```python
from build123d import *

# Parameters (mm, degrees)
BOSS_EXTRUDE1_DEPTH = 2.6
SKETCH3_R           = 1.7
SKETCH3_R_2         = 0.75
BOSS_EXTRUDE2_DEPTH = 4.4
CUT_EXTRUDE1_DEPTH  = 48.070691518
LPATTERN1_COUNT     = 6
LPATTERN1_PITCH     = 8
SKETCH4_R           = 1.95
CUT_EXTRUDE2_DEPTH  = 47.754785851
SKETCH6_W           = 2.6
SKETCH6_H           = 3.6
SKETCH6_W_2         = 4.3
SKETCH6_H_2         = 2.6
BOSS_EXTRUDE4_DEPTH = 1.8
SKETCH7_W           = 2.6
SKETCH7_H           = 1.6
SKETCH7_W_2         = 1.6
SKETCH7_H_2         = 2.6
BOSS_EXTRUDE5_DEPTH = 2
BOSS_EXTRUDE6_START = -2.6
BOSS_EXTRUDE6_DEPTH = 2.6
SKETCH9_R           = 8.5
SKETCH9_R_2         = 4.3
BOSS_EXTRUDE7_DEPTH = 4
SKETCH12_R          = 0.95
CUT_EXTRUDE3_DEPTH  = 4
SKETCH13_W          = 11.452487144
SKETCH13_H          = 18.554951014
SKETCH13_W_2        = 15.080629567
SKETCH13_H_2        = 21.043729538
CUT_EXTRUDE4_DEPTH  = 4
FILLET1_R           = 1
FILLET2_R           = 1


with BuildPart() as part:
    # Sketch1 → Boss-Extrude1 (new body)
    with BuildSketch(Plane(origin=(0, 0, 0), x_dir=(1, 0, 0), z_dir=(0, 1, 0))):
        with BuildLine():
            Line((-33.9, -30.8), (30.9, -30.8))
            ThreePointArc((30.9, -30.8), (33.728427125, -29.628427125), (34.9, -26.8))
            Line((34.9, -26.8), (34.9, 26.8))
            ThreePointArc((34.9, 26.8), (33.728427125, 29.628427125), (30.9, 30.8))
            Line((30.9, 30.8), (-33.9, 30.8))
            ThreePointArc((-33.9, 30.8), (-34.607106781, 30.507106781), (-34.9, 29.8))
            Line((-34.9, 29.8), (-34.9, -29.8))
            ThreePointArc((-34.9, -29.8), (-34.607106781, -30.507106781), (-33.9, -30.8))
        make_face()
    extrude(amount=BOSS_EXTRUDE1_DEPTH)

    # Sketch3 → Boss-Extrude2 (add)
    # profile 1 of 4: a face of its own
    with BuildSketch(Plane.XZ):
        with Locations(Location((-28.9, 16, 0), (0, 0, 270))):
            Circle(SKETCH3_R)
        with Locations(Location((-28.9, 16, 0), (0, 0, 270))):
            Circle(SKETCH3_R_2, mode=Mode.SUBTRACT)
    # profile 2 of 4: a face of its own
    with BuildSketch(Plane.XZ):
        with Locations(Location((3.1, 16, 0), (0, 0, 270))):
            Circle(SKETCH3_R)
        with Locations(Location((3.1, 16, 0), (0, 0, 270))):
            Circle(SKETCH3_R_2, mode=Mode.SUBTRACT)
    # profile 3 of 4: a face of its own
    with BuildSketch(Plane.XZ):
        with Locations(Location((-28.9, -16, 0), (0, 0, 270))):
            Circle(SKETCH3_R)
        with Locations(Location((-28.9, -16, 0), (0, 0, 270))):
            Circle(SKETCH3_R_2, mode=Mode.SUBTRACT)
    # profile 4 of 4: a face of its own
    with BuildSketch(Plane.XZ):
        with Locations(Location((3.1, -16, 0), (0, 0, 270))):
            Circle(SKETCH3_R)
        with Locations(Location((3.1, -16, 0), (0, 0, 270))):
            Circle(SKETCH3_R_2, mode=Mode.SUBTRACT)
    extrude(amount=BOSS_EXTRUDE2_DEPTH)

    # Sketch2 → Cut-Extrude1 (cut, through all)
    with BuildSketch(Plane(origin=(0, 2.6, 0), x_dir=(1, 0, 0), z_dir=(0, 1, 0))):
        with BuildLine():
            Line((28.9, -21.5), (6.1, -21.5))
            ThreePointArc((6.1, -21.5), (4.6, -20), (6.1, -18.5))
            Line((6.1, -18.5), (28.9, -18.5))
            ThreePointArc((28.9, -18.5), (30.4, -20), (28.9, -21.5))
        make_face()
        with BuildLine():
            Line((0.1, -21.5), (-25.9, -21.5))
            ThreePointArc((-25.9, -21.5), (-27.4, -20), (-25.9, -18.5))
            Line((-25.9, -18.5), (0.1, -18.5))
            ThreePointArc((0.1, -18.5), (1.6, -20), (0.1, -21.5))
        make_face()
    cut_extrude1 = extrude(amount=-CUT_EXTRUDE1_DEPTH, mode=Mode.SUBTRACT)

    # LPattern1: Cut-Extrude1 ×6
    with Locations(*[(0, 0, -i * LPATTERN1_PITCH) for i in range(1, LPATTERN1_COUNT)]):
        add(cut_extrude1, mode=Mode.SUBTRACT)

    # Sketch4 → Cut-Extrude2 (cut, through all)
    with BuildSketch(Plane.XZ):
        with Locations(Location((27.9, 0, 0), (0, 0, 270))):
            Circle(SKETCH4_R)
        with BuildLine():
            Line((-28.9, 25), (28.9, 25))
            ThreePointArc((28.9, 25), (29.9, 24), (28.9, 23))
            Line((28.9, 23), (-28.9, 23))
            ThreePointArc((-28.9, 23), (-29.9, 24), (-28.9, 25))
        make_face()
        with BuildLine():
            Line((-24.9, 17), (-0.9, 17))
            ThreePointArc((-0.9, 17), (0.1, 16), (-0.9, 15))
            Line((-0.9, 15), (-24.9, 15))
            ThreePointArc((-24.9, 15), (-25.9, 16), (-24.9, 17))
        make_face()
        with BuildLine():
            Line((7.1, 17), (28.9, 17))
            ThreePointArc((28.9, 17), (29.9, 16), (28.9, 15))
            Line((28.9, 15), (7.1, 15))
            ThreePointArc((7.1, 15), (6.1, 16), (7.1, 17))
        make_face()
        with BuildLine():
            Line((-24.9, -15), (-0.9, -15))
            ThreePointArc((-0.9, -15), (0.1, -16), (-0.9, -17))
            Line((-0.9, -17), (-24.9, -17))
            ThreePointArc((-24.9, -17), (-25.9, -16), (-24.9, -15))
        make_face()
        with BuildLine():
            Line((7.1, -15), (28.9, -15))
            ThreePointArc((28.9, -15), (29.9, -16), (28.9, -17))
            Line((28.9, -17), (7.1, -17))
            ThreePointArc((7.1, -17), (6.1, -16), (7.1, -15))
        make_face()
        with BuildLine():
            Line((-28.9, -23), (28.9, -23))
            ThreePointArc((28.9, -23), (29.9, -24), (28.9, -25))
            Line((28.9, -25), (-28.9, -25))
            ThreePointArc((-28.9, -25), (-29.9, -24), (-28.9, -23))
        make_face()
        with BuildLine():
            Line((-28.9, 9), (18.9, 9))
            ThreePointArc((18.9, 9), (19.9, 8), (18.9, 7))
            Line((18.9, 7), (-28.9, 7))
            ThreePointArc((-28.9, 7), (-29.9, 8), (-28.9, 9))
        make_face()
        with BuildLine():
            Line((18.9, -1), (-28.9, -1))
            ThreePointArc((-28.9, -1), (-29.9, 0), (-28.9, 1))
            Line((-28.9, 1), (18.9, 1))
            ThreePointArc((18.9, 1), (19.9, 0), (18.9, -1))
        make_face()
        with BuildLine():
            Line((-28.9, -7), (18.9, -7))
            ThreePointArc((18.9, -7), (19.9, -8), (18.9, -9))
            Line((18.9, -9), (-28.9, -9))
            ThreePointArc((-28.9, -9), (-29.9, -8), (-28.9, -7))
        make_face()
    extrude(amount=-CUT_EXTRUDE2_DEPTH, mode=Mode.SUBTRACT)

    # Sketch6 → Boss-Extrude4 (add)
    with BuildSketch(Plane.XZ):
        with Locations((-21.4, 29)):
            Rectangle(SKETCH6_W, SKETCH6_H)
        with Locations((-21.4, -29)):
            Rectangle(SKETCH6_W, SKETCH6_H)
        with Locations((32.75, 17.25)):
            Rectangle(SKETCH6_W_2, SKETCH6_H_2)
        with Locations((32.75, -17.25)):
            Rectangle(SKETCH6_W_2, SKETCH6_H_2)
    extrude(amount=BOSS_EXTRUDE4_DEPTH)

    # Sketch7 → Boss-Extrude5 (add)
    with BuildSketch(Plane.XZ.offset(1.8)):
        with Locations((-21.4, 28)):
            Rectangle(SKETCH7_W, SKETCH7_H)
        with Locations((31.4, 17.25)):
            Rectangle(SKETCH7_W_2, SKETCH7_H_2)
        with Locations((31.4, -17.25)):
            Rectangle(SKETCH7_W_2, SKETCH7_H_2)
        with Locations((-21.4, -28)):
            Rectangle(SKETCH7_W, SKETCH7_H)
    extrude(amount=BOSS_EXTRUDE5_DEPTH)

    # Sketch8 → Boss-Extrude6 (add)
    with BuildSketch(Plane.XZ.offset(BOSS_EXTRUDE6_START)):
        with BuildLine():
            Line((28.9, -5.5), (18.9, -5.5))
            ThreePointArc((18.9, -5.5), (20.4, -4), (18.9, -2.5))
            Line((18.9, -2.5), (28.9, -2.5))
            ThreePointArc((28.9, -2.5), (30.4, -4), (28.9, -5.5))
        make_face()
        with BuildLine():
            Line((28.9, 2.5), (18.9, 2.5))
            ThreePointArc((18.9, 2.5), (20.4, 4), (18.9, 5.5))
            Line((18.9, 5.5), (28.9, 5.5))
            ThreePointArc((28.9, 5.5), (30.4, 4), (28.9, 2.5))
        make_face()
    extrude(amount=BOSS_EXTRUDE6_DEPTH)

    # Sketch9 → Boss-Extrude7 (add)
    with BuildSketch(Plane.XZ):
        with Locations(Location((27.9, 0, 0), (0, 0, 34.56032178))):
            Circle(SKETCH9_R)
        with Locations(Location((27.9, 0, 0), (0, 0, 270))):
            Circle(SKETCH9_R_2, mode=Mode.SUBTRACT)
    extrude(amount=BOSS_EXTRUDE7_DEPTH)

    # Sketch12 → Cut-Extrude3 (cut)
    with BuildSketch(Plane.XZ.offset(4)):
        with Locations(Location((27.9, 6.15, 0), (0, 0, 270))):
            Circle(SKETCH12_R)
        with Locations(Location((27.9, -6.15, 0), (0, 0, 270))):
            Circle(SKETCH12_R)
    extrude(amount=-CUT_EXTRUDE3_DEPTH, mode=Mode.SUBTRACT)

    # Sketch13 → Cut-Extrude4 (cut)
    with BuildSketch(Plane.XZ.offset(4)):
        with Locations((36.626243572, 0.035430506)):
            Rectangle(SKETCH13_W, SKETCH13_H)
        with Locations((17.359685217, 0.379129228)):
            Rectangle(SKETCH13_W_2, SKETCH13_H_2)
    extrude(amount=-CUT_EXTRUDE4_DEPTH, mode=Mode.SUBTRACT)

    # Fillet1
    fillet1_edges = [part.edges().sort_by_distance(p)[0] for p in [
        (24.9, -2, 3.08058436),
        (24.9, -2, -3.08058436),
        (30.9, -2, -3.08058436),
        (30.9, -2, 3.08058436),
    ]]
    fillet(fillet1_edges, radius=FILLET1_R)

    # Fillet2
    fillet2_edges = [part.edges().sort_by_distance(p)[0] for p in [
        (30.9, -2, 7.95298686),
        (30.9, -2, -7.95298686),
        (24.9, -2, -7.95298686),
        (24.9, -2, 7.95298686),
    ]]
    fillet(fillet2_edges, radius=FILLET2_R)


solid = part.part
```
Work out the finished part from the listing and answer in its coordinate system (mm). A direction names the side the tool comes from. Coordinates: 2 decimals unless noted, no trailing zeros. Write each loop counter-clockwise with the first axis right and the second up, starting at its lowest first coordinate (ties: lowest second). Pieces come first, ordered by that corner, then holes.
Q1. A cutting plane is placed at C-C, the plane y = 1.5. State how many separate pieces and enclosed holes the cut face has, then the cut area to 3 significant figures.
Q2. Find the intervals of material crossed by line 1 (X direction, y = 1.4, z = 0); line 2 (X direction, y = -3, z = -16); line 3 (X direction, y = -1.05, z = 16), in increasing order.
Q3. Determine the mould class of faces 1 (the face through (24.9, -2, -6)), 2 (the face through (-21, -2, -27.2)), 3 (the face through (-13, 1, -5.5)), 4 (the face through (17, 1, -21.5)) for opening direction X: released by +X, released by -X, zero draft, split by the parting line, or undercut.
Q4. Each of these flat-tipped pins is pushed along its axis until it touches: pin 1 Ø10 at (x, z) = (-20, -21.5) entering from -Y; pin 2 Ø1 at (x, y) = (-21, -2.5) entering from -Z; pin 3 Ø1.9 at (y, z) = (-2.5, 6.5) entering from +X. Where does it stop, or does it pass through?
Q5. Which of the six approach directions +Z, -Z, +X, -X, +Y, -Y give full straight-line access (tool end or side, diameter ignored) to faces 5 (the face through (32.2, -3, -17)), 6 (the face through (3, 0, 16)), 7 (the face through (-27.4, 1.3, 4)), 8 (the face through (30.6, -2, -17))?
Q6. A cutting plane is placed at B-B, the plane z = -20. Give the vertices of the cut face in (x, y), then the cut area to 3 significant figures.
Q7. A cutting plane is placed at A-A, the plane z = 24. Give the vertices of the cut face in (x, y).
Findings below:
1. separate pieces: 1
1. enclosed holes: 22
1. area: 2,650 mm2
2. line 1: x = -34.9 to -29.9, 19.9 to 25.95, 29.85 to 34.9
2. line 2: x = -30.6 to -29.65, -28.15 to -27.2, 1.4 to 2.35, 3.85 to 4.8, 30.6 to 32.2
2. line 3: x = -30.6 to -29.65, -28.15 to -27.2, 1.4 to 2.35, 3.85 to 4.8, 30.6 to 34.9
3. face 1: released by -X
3. face 2: zero draft
3. face 3: undercut
3. face 4: undercut
4. pin 1: stops at y = 0
4. pin 2: stops at z = -28.8
4. pin 3: stops at x = 30.9
5. face 5: +Z, -Z, +X, -Y
5. face 6: -Y
5. face 7: +Y, -Y
5. face 8: -Z, -Y
6. outline: (-34.9, 0) - (-27.4, 0) - (-27.4, 2.6) - (-34.9, 2.6) - close; (1.6, 0) - (4.6, 0) - (4.6, 2.6) - (1.6, 2.6) - close; (30.4, 0) - (34.9, 0) - (34.9, 2.6) - (30.4, 2.6) - close
6. area: 39.0 mm2
7. outline: (-34.9, 0) - (-29.9, 0) - (-29.9, 2.6) - (-34.9, 2.6) - close; (29.9, 0) - (34.9, 0) - (34.9, 2.6) - (29.9, 2.6) - close
